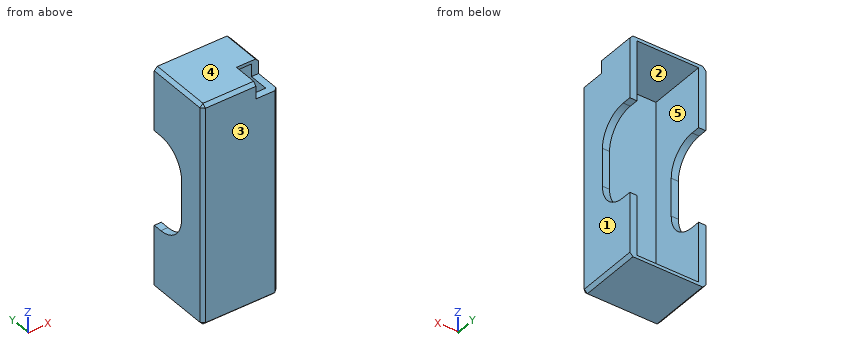
```python
from build123d import *

# Parameters (mm, degrees)
SKETCH1_W               = 24
SKETCH1_H               = 70
BOSS_EXTRUDE1_DEPTH     = 20.7
SKETCH2_W               = 19.5
SKETCH2_H               = 68
CUT_EXTRUDE1_DEPTH      = 18.45
CUT_EXTRUDE2_DEPTH      = 48.217475578
CUT_EXTRUDE2_DEPTH_BACK = 48.217475578
SKETCH4_W               = 30
SKETCH4_H               = 11.85
FILLET1_R               = 9
SKETCH5_W               = 7
SKETCH5_H               = 8.41
CUT_EXTRUDE3_DEPTH      = 5
CHAMFER1_SIZE           = 1


with BuildPart() as part:
    # Sketch1 → Boss-Extrude1 (new body)
    with BuildSketch(Plane(origin=(0, 0, 0), x_dir=(1, 0, 0), z_dir=(0, 1, 0))):
        Rectangle(SKETCH1_W, SKETCH1_H)
    extrude(amount=BOSS_EXTRUDE1_DEPTH)

    # Sketch2 → Cut-Extrude1 (cut)
    with BuildSketch(Plane(origin=(0, 20.7, 0), x_dir=(1, 0, 0), z_dir=(0, 1, 0))):
        Rectangle(SKETCH2_W, SKETCH2_H)
    extrude(amount=-CUT_EXTRUDE1_DEPTH, mode=Mode.SUBTRACT)

    # Sketch4 → Cut-Extrude2 (cut, two sides: drawn at the far end of the back side and taken through both)
    with BuildSketch(Plane.ZY.offset(12).offset(-CUT_EXTRUDE2_DEPTH_BACK)):
        with Locations((0, 14.775)):
            Rectangle(SKETCH4_W, SKETCH4_H)
    extrude(amount=CUT_EXTRUDE2_DEPTH + CUT_EXTRUDE2_DEPTH_BACK, mode=Mode.SUBTRACT)

    # Fillet1
    fillet1_edges = [part.edges().sort_by_distance(p)[0] for p in [
        (-10.875, 8.85, -15),
        (10.875, 8.85, -15),
        (-10.875, 8.85, 15),
        (10.875, 8.85, 15),
    ]]
    fillet(fillet1_edges, radius=FILLET1_R)

    # Sketch5 → Cut-Extrude3 (cut)
    with BuildSketch(Plane.XY.offset(35)):
        with Locations((8.5, 4.205)):
            Rectangle(SKETCH5_W, SKETCH5_H)
    extrude(amount=-CUT_EXTRUDE3_DEPTH, mode=Mode.SUBTRACT)

    # Chamfer1
    chamfer1_edges = [part.edges().sort_by_distance(p)[0] for p in [
        (0, 0, -35),
        (-3.5, 0, 35),
        (-12, 0, 0),
        (-12, 10.35, -35),
        (12, 10.35, -35),
        (12, 14.555, 35),
        (-12, 10.35, 35),
        (12, 0, -2.5),
    ]]
    chamfer(chamfer1_edges, length=CHAMFER1_SIZE)


solid = part.part
```
Source: CAD feature listing. Evaluate the final solid. Frame: model axes, mm. Face numbers are marked on the shaded views. A direction names the side the tool comes from. Round coordinates to 2 decimals unless told otherwise and drop trailing zeros. Loops run counter-clockwise (first coordinate to the right, second up) from the corner with the lowest first, then second, coordinate; pieces in that order, holes last.
(1) Material intervals for probe 1 along X at (y, z) = (18.75, 26.5); probe 2 along Z at (x, y) = (3.5, 3.5); probe 3 along Z at (x, y) = (9.25, 5), sorted ascending.
From the geometry:
probe 1: x = -12 to -9.75, 9.75 to 12
probe 2: z = -35 to -34, 34 to 35
probe 3: z = -35 to -34
(2) Access query for the marked faces 4 and 5. Directions: +Z, -Z, +X, -X, +Y, -Y. A direction counts if a zero-diameter tool reaches every point of the face in a straight line with its end or side. Return the directions, or none.
From the geometry:
face 4: +Z, +X, -X, +Y, -Y
face 5: +Y
(3) Section query B-B (z = 5). Output: boundary loops of the cut face in (x, y).
From the geometry:
outline: (-12, 1) - (-11, 0) - (11, 0) - (12, 1) - (12, 8.85) - (9.75, 8.85) - (9.75, 2.25) - (-9.75, 2.25) - (-9.75, 8.85) - (-12, 8.85) - close
(4) Contact query for flat-ended pins moving along their axis: pin 1 Ø1.8 at (x, z) = (11.5, -3) entering from +Y; pin 2 Ø4 at (y, z) = (5.5, 31.5) entering from +X; pin 3 Ø2 at (x, y) = (10, 4.5) entering from +Z; pin 4 Ø10 at (x, z) = (4.5, 13) entering from +Y. Output: stop coordinate, or through.
From the geometry:
pin 1: stops at y = 8.85
pin 2: stops at x = 12
pin 3: stops at z = 30
pin 4: stops at y = 2.25
(5) Pull-direction query (X, two-part tool) for the marked faces 1, 2 and 3; classes: +X half, -X half, draft (parallel to the pull), parting line (faces both ways), or undercut.
From the geometry:
face 1: +X half
face 2: undercut
face 3: draft
(6) Section query A-A (y = 18.75). Output: boundary loops of the cut face in (x, z), and give its area (3 significant figures).
From the geometry:
outline: (-12, -34) - (-11, -35) - (11, -35) - (12, -34) - (12, -15) - (9.75, -15) - (9.75, -34) - (-9.75, -34) - (-9.75, -15) - (-12, -15) - close; (-12, 15) - (-9.75, 15) - (-9.75, 34) - (9.75, 34) - (9.75, 15) - (12, 15) - (12, 34) - (11, 35) - (-11, 35) - (-12, 34) - close
area: 217 mm2
(7) Section query C-C (x = 1.5). Output: boundary loops of the cut face in (y, z).
From the geometry:
outline: (0, -34) - (1, -35) - (20.7, -35) - (20.7, -34) - (2.25, -34) - (2.25, 34) - (20.7, 34) - (20.7, 35) - (1, 35) - (0, 34) - close
(8) Section query D-D (y = 7.5). Output: boundary loops of the cut face in (x, z), and give its area (4 significant figures).
From the geometry:
outline: (-12, -34) - (-11, -35) - (11, -35) - (12, -34) - (12, 30) - (9.75, 30) - (9.75, -34) - (-9.75, -34) - (-9.75, 34) - (5, 34) - (5, 35) - (-11, 35) - (-12, 34) - close
area: 336.5 mm2
